from build123d import *

# Parameters (mm, degrees)
F1_DEPTH    = 45.212
F2_T1_DEPTH = 97.7563484187


# Not quite as in the source:
# - a fillet or chamfer that OpenCascade refuses, or shapes differently, is made with other operations: its cross-section is extruded or revolved along the edge and cut away or added


with BuildPart() as f1:
    # F0 (on Front) → F1 (new body, symmetric)
    with BuildSketch(Plane.XZ):
        Polygon((53.9703455338, -18.609975213), (43.1018840651, 37.4347026768), (-10.8684614687, 56.0446778898), (-53.9703455338, 18.609975213), (-43.1018840651, -37.4347026768), (10.8684614687, -56.0446778898), align=None)
    extrude(amount=F1_DEPTH, both=True)

    # F2: fillet of radius 2.54 on 6 edges, made by hand

    # F2_s2 → F2_t1 (cut)
    with BuildSketch(Plane.XZ.offset(-48.8781742094)):
        with BuildLine():
            add(Edge.make_bspline(
                [(-11.9756422622, 55.0830729689), (-10.8684614687, 56.0446778898), (-9.4820967821, 55.5666336564)],
                knots=[0, 0, 0, 1, 1, 1], degree=2, weights=[1, 1, 1]))
            Line((-9.4820967821, 55.5666336564), (-10.8684614687, 56.0446778898))
            Line((-10.8684614687, 56.0446778898), (-11.9756422622, 55.0830729689))
        make_face()
        with BuildLine():
            add(Edge.make_bspline(
                [(43.3810679582, 35.9950535226), (43.1018840651, 37.4347026768), (41.7155193785, 37.9127469102)],
                knots=[0, 0, 0, 1, 1, 1], degree=2, weights=[1, 1, 1]))
            Line((41.7155193785, 37.9127469102), (43.1018840651, 37.4347026768))
            Line((43.1018840651, 37.4347026768), (43.3810679582, 35.9950535226))
        make_face()
        with BuildLine():
            add(Edge.make_bspline(
                [(-53.6911616407, 17.1703260588), (-53.9703455338, 18.609975213), (-52.8631647403, 19.5715801338)],
                knots=[0, 0, 0, 1, 1, 1], degree=2, weights=[1, 1, 1]))
            Line((-52.8631647403, 19.5715801338), (-53.9703455338, 18.609975213))
            Line((-53.9703455338, 18.609975213), (-53.6911616407, 17.1703260588))
        make_face()
        with BuildLine():
            add(Edge.make_bspline(
                [(-41.7155193785, -37.9127469102), (-43.1018840651, -37.4347026768), (-43.3810679582, -35.9950535226)],
                knots=[0, 0, 0, 1, 1, 1], degree=2, weights=[1, 1, 1]))
            Line((-43.3810679582, -35.9950535226), (-43.1018840651, -37.4347026768))
            Line((-43.1018840651, -37.4347026768), (-41.7155193785, -37.9127469102))
        make_face()
        with BuildLine():
            add(Edge.make_bspline(
                [(11.9756422622, -55.0830729689), (10.8684614687, -56.0446778898), (9.4820967821, -55.5666336564)],
                knots=[0, 0, 0, 1, 1, 1], degree=2, weights=[1, 1, 1]))
            Line((9.4820967821, -55.5666336564), (10.8684614687, -56.0446778898))
            Line((10.8684614687, -56.0446778898), (11.9756422622, -55.0830729689))
        make_face()
        with BuildLine():
            add(Edge.make_bspline(
                [(53.6911616407, -17.1703260588), (53.9703455338, -18.609975213), (52.8631647403, -19.5715801338)],
                knots=[0, 0, 0, 1, 1, 1], degree=2, weights=[1, 1, 1]))
            Line((52.8631647403, -19.5715801338), (53.9703455338, -18.609975213))
            Line((53.9703455338, -18.609975213), (53.6911616407, -17.1703260588))
        make_face()
    extrude(amount=F2_T1_DEPTH, mode=Mode.SUBTRACT)


solid = f1.part
The model under review builds one solid part; all positions refer to its coordinate system, in mm. Coordinates: 2 decimals unless noted, no trailing zeros. Loops run counter-clockwise (first coordinate to the right, second up) from the corner with the lowest first, then second, coordinate; pieces in that order, holes last.
(1) Insertion check: P1, Ø1, axis at x = 0, y = -36, coming from the +Z side; P2, Ø3, axis at x = -33, y = -19.5, coming from the -Z side; P3, Ø5, axis at x = 25, y = -5, coming from the +Z side; P4, Ø8, axis at y = -3, z = 14, coming from the -X side. Each pin has a flat end and moves straight along its axis. Give the tip position at first contact, or say it passes through.
Determined:
P1: stops at z = 52.47
P2: stops at z = -41.44
P3: stops at z = 44.54
P4: stops at x = -53.75
(2) Consider section B-B, the plane x = 32. Give the boundary of the cut face in (y, z).
Determined:
outline: (-45.21, -37.69) - (45.21, -37.69) - (45.21, 41.26) - (-45.21, 41.26) - close
(3) Draft analysis for pull direction Y (two halves, no side actions). For faces 1 (the flat face through (-16.475, -0.633, -46.616)), 2 (the flat face through (-1, -45.212, 1)), 3 (the flat face through (-1, 45.212, 1)), state which applies: +Y half, -Y half, draft (parallel to the pull), parting line (faces both ways), or undercut.
Determined:
face 1: draft
face 2: -Y half
face 3: +Y half
(4) Wall thickness on L1, parallel to X at y = -19.5, z = -23.5; L2, parallel to X at y = -27, z = -25; L3, parallel to Z at x = 6, y = -35: over which ranges is each line inside the solid? List them lowest first.
Determined:
L1: x = -45.8 to 48.34
L2: x = -45.51 to 46.61
L3: z = -54.37 to 50.23
(5) Consider section A-A, the plane z = 45.5. Give the boundary of the cut face in (x, y).
Determined:
outline: (-23.01, -45.21) - (19.71, -45.21) - (19.71, 45.21) - (-23.01, 45.21) - close
